Read the model definition and answer for the solid it produces. Units are mm, in the model's axes. A direction names the side the tool comes from. Coordinates: 2 decimals unless noted, no trailing zeros. Order: outer loops, then holes, each group sorted by start corner. A loop starts at its lowest first (then second) coordinate and runs counter-clockwise, first axis right, second up.
Autodesk Inventor part; units mm, degrees
ref_plane "YZ Plane" through (0, 0, 0) normal (1, 0, 0) x (0, 1, 0)
ref_plane "XZ Plane" through (0, 0, 0) normal (0, 1, 0) x (-1, 0, 0)
ref_plane "XY Plane" through (0, 0, 0) normal (0, 0, 1) x (1, 0, 0)
sketch "Sketch1" plane through (0, 0, 0) normal (0, 1, 0) x (-1, 0, 0)
  line L0 (0, 0) -> (55, 0)
  line L1 (55, 0) -> (55, -55)
  line L2 (55, -55) -> (0, -55)
  line L3 (0, -55) -> (0, 0)
  line L4 (55, -27.5) -> (0, -27.5) construction
  line L5 (27.5, -55) -> (27.5, 0) construction
  line L6 (20.3868, -55) -> (34.6132, -55)
  line L7 (34.6842, -50) -> (21.2609, -50)
  line L8 (50, -17.5) -> (50, -33.6438)
  line L9 (55, -34.6132) -> (55, -20.3868)
  line L10 (5, -18.3051) -> (5, -36.8563)
  line L11 (0, -34.6132) -> (0, -20.3868)
  line L12 (20.3868, 0) -> (34.6132, 0)
  line L13 (37.7365, -5) -> (17.5, -5)
  line L14 (55, -34.6132) -> (50, -37.5)
  line L15 (50, -37.5) -> (50, -33.6438)
  line L16 (55, -20.3868) -> (50, -17.5)
  line L17 (34.6842, -50) -> (37.5, -50)
  line L18 (37.5, -50) -> (34.6132, -55)
  line L19 (21.2609, -50) -> (17.5, -50)
  line L20 (17.5, -50) -> (20.3868, -55)
  line L21 (0, -34.6132) -> (5, -37.5)
  line L22 (5, -37.5) -> (5, -36.8563)
  line L23 (0, -20.3868) -> (5, -17.5)
  line L24 (5, -17.5) -> (5, -18.3051)
  line L25 (20.3868, 0) -> (17.5, -5)
  line L26 (34.6132, 0) -> (37.5, -5)
  line L27 (37.5, -5) -> (37.7365, -5)
  line L28 (55, -47.5) -> (47.5, -55)
  line L29 (55, -7.5) -> (47.5, 0)
  line L30 (7.5, -55) -> (0, -47.5)
  line L31 (7.5, 0) -> (0, -7.5)
  line L32 (55, 0) -> (0, 0)
  line L33 (0, 0) -> (0, -55)
  line L34 (0, -55) -> (55, -55)
  line L35 (55, -55) -> (55, 0)
  dimension "d0" = 55
  dimension "d1" = 55
  dimension "d4" = 5
  dimension "d5" = 5
  dimension "d6" = 60
  dimension "d9" = 60
  dimension "d10" = 60
  dimension "d13" = 20
  dimension "d14" = 10
  dimension "d15" = 60
  dimension "d16" = 5
  dimension "d18" = 60
  dimension "d19" = 5
  dimension "d20" = 20
  dimension "d21" = 10
  dimension "d22" = 10
  dimension "d23" = 20
  dimension "d24" = 20
  dimension "d25" = 10
  dimension "d26" = 7.5
  dimension "d27" = 7.5
  dimension "d28" = 7.5
  dimension "d29" = 7.5
  dimension "d30" = 7.5
  dimension "d31" = 7.5
extrude "Extrusion1" add sketch "Sketch1" along normal blind 5 contours L0 L25 L13 L26 L29 L1 L16 L8 L15 L14 L28 L2 L18 L17 L7 L19 L20 L30 L3 L21 L22 L10 L24 L23 L31
extrude "Extrusion2" add sketch "Sketch1" along normal blind 60 draft 1.75 contours L0 L31 L3 | L0 L1 L29 | L30 L2 L3 | L1 L2 L28
fillet "Fillet1" radius 5 4 edges at (-3.858, 5, -51.142) (-3.858, 5, -3.858) (-51.142, 5, -51.142) (-51.142, 5, -3.858)
equation "\"d0\" = side_length"
equation "\"d1\" = side_length"
equation "\"d4\" = dovetail_depth"
equation "\"d5\" = dovetail_depth"
equation "\"d13\" = dovetail_max_length"
equation "\"d14\" = 0.5 * dovetail_max_length"
equation "\"d16\" = dovetail_depth"
equation "\"d19\" = dovetail_depth"
equation "\"d20\" = dovetail_max_length"
equation "\"d21\" = 0.5 * dovetail_max_length"
equation "\"d22\" = 0.5 * dovetail_max_length"
equation "\"d23\" = dovetail_max_length"
equation "\"d24\" = dovetail_max_length"
equation "\"d25\" = 0.5 * dovetail_max_length"
equation "\"d26\" = claw_wall_side_length"
equation "\"d27\" = claw_wall_side_length"
equation "\"d28\" = claw_wall_side_length"
equation "\"d29\" = claw_wall_side_length"
equation "\"d30\" = claw_wall_side_length"
equation "\"d31\" = claw_wall_side_length"
equation "\"side_length\" = 55"
equation "\"dovetail_depth\" = 5"
equation "\"dovetail_max_length\" = 20"
equation "\"claw_wall_side_length\" = 7.5"
equation "\"band_notch_height\" = 45"
properties part number "Duck_Holder"
1) A cutting plane is placed at A-A, the plane y = 34.5. Determine the outline of the cut face in (x, z), and give its area (3 significant figures).
A:
outline: (-56.05, -56.05) - (-44.96, -56.05) - (-56.05, -44.96) - close; (-56.05, -10.04) - (-44.96, 1.05) - (-56.05, 1.05) - close; (-10.04, -56.05) - (1.05, -56.05) - (1.05, -44.96) - close; (-10.04, 1.05) - (1.05, -10.04) - (1.05, 1.05) - close
area: 246 mm2
2) Determine the mould class of faces 1 (the flat face through (-55, 3, -12)), 2 (the flat face through (-27, 0, -27)) for opening direction Z: pulls with the +Z half, pulls with the -Z half, needs draft (parallel to the pull), parting line crosses it, or undercut.
A:
face 1: undercut
face 2: needs draft
3) A cutting plane is placed at C-C, the plane y = 52.5. Determine the outline of the cut face in (x, z).
A:
outline: (-56.6, -56.6) - (-43.63, -56.6) - (-56.6, -43.63) - close; (-56.6, -11.37) - (-43.63, 1.6) - (-56.6, 1.6) - close; (-11.37, -56.6) - (1.6, -56.6) - (1.6, -43.63) - close; (-11.37, 1.6) - (1.6, -11.37) - (1.6, 1.6) - close
4) Which of the six approach directions +Z, -Z, +X, -X, +Y, -Y give full straight-line access (tool end or side, diameter ignored) to faces 3 (the flat face through (-2.47, 2.46, -36.04)), 4 (the flat face through (-27, 5, -27)), 5 (the flat face through (-3, 60, -3)), 6 (the cylindrical face through (-49.632, 5.906, -5.578))?
A:
face 3: +Y, -Y
face 4: +Y
face 5: +Z, -Z, +X, -X, +Y
face 6: none
5) A cutting plane is placed at B-B, the plane x = -33.5. Determine the outline of the cut face in (y, z).
A:
outline: (0, -50) - (5, -50) - (5, -5) - (0, -5) - close
6) A cutting plane is placed at D-D, the plane z = -16. Determine the outline of the cut face in (x, y), and give its area (3 significant figures).
A:
outline: (-55, 0) - (0, 0) - (0, 5) - (-55, 5) - close
area: 275 mm2
7) Flat-ended cylindrical pins translate along their axes: pin 1 Ø1.5 at (x, y) = (-27.5, 1.5) entering from +Z; pin 2 Ø6 at (y, z) = (38, -6.5) entering from +X; pin 3 Ø1.5 at (y, z) = (2.5, -30) entering from +X. Find the tip coordinate at first contact, or state that the pin passes through.
A:
pin 1: stops at z = -5
pin 2: stops at x = 1.25
pin 3: stops at x = -5
8) Straight lines are drawn through the part: line 1 (X direction, y = 50, z = -8); line 2 (Z direction, x = -24, y = 4.5); line 3 (Y direction, x = -16, z = -20). For each, find the intervals that lie inside material, in ascending order.
A:
line 1: x = -56.53 to -53.34, -1.66 to 1.53
line 2: z = -50 to -5
line 3: y = 0 to 5
